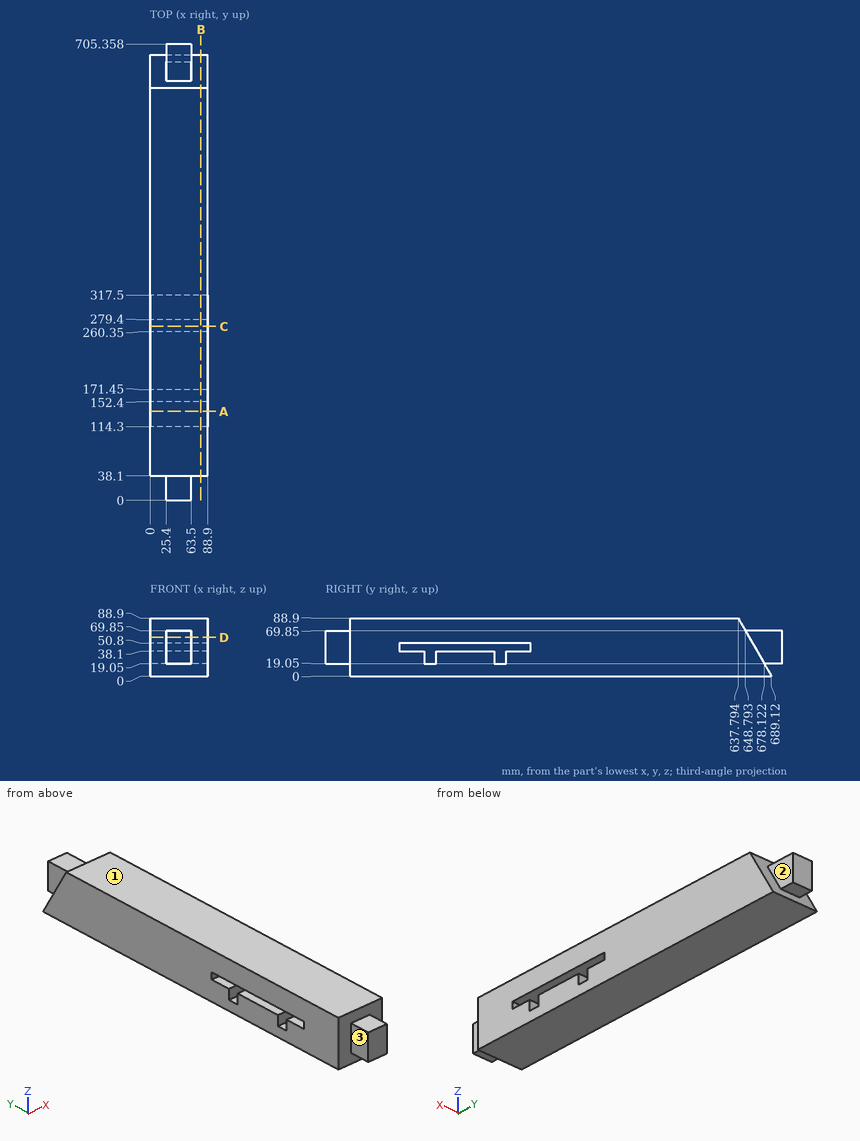
Geometry check sheet. Reference: drawing and pictorial views, mm from the part's lowest x, y, z. A direction names the side the tool comes from. Round coordinates to 2 decimals unless told otherwise and drop trailing zeros. Write each loop counter-clockwise with the first axis right and the second up, starting at its lowest first coordinate (ties: lowest second). Pieces come first, ordered by that corner, then holes. Notation, with made-up numbers: (-5.75, 34) -> (46.25, 34) arc R10 ccw to (46.25, 51) -> close; hole circle Ø4 at (-35, 2.5). An arc over 180 degrees is marked (long way). Put each result on its own line as item: value.
1) Cross-section at A-A, the plane y = 137.5. Enter the section's corners in (x, z), plus the area to 3 significant figures.
Recorded:
outline: (0, 0) -> (88.9, 0) -> (88.9, 38.1) -> (0, 38.1) -> close; (0, 50.8) -> (88.9, 50.8) -> (88.9, 88.9) -> (0, 88.9) -> close
area: 6,770 mm2
2) Cross-section at D-D, the plane z = 59.5. Enter the section's corners in (x, y).
Recorded:
outline: (0, 38.1) -> (25.4, 38.1) -> (25.4, 0) -> (63.5, 0) -> (63.5, 38.1) -> (88.9, 38.1) -> (88.9, 654.77) -> (63.5, 654.77) -> (63.5, 705.36) -> (25.4, 705.36) -> (25.4, 654.77) -> (0, 654.77) -> close
3) Cross-section at B-B, the plane x = 78.5. Enter the section's corners in (y, z).
Recorded:
outline: (38.1, 0) -> (689.12, 0) -> (637.79, 88.9) -> (38.1, 88.9) -> close; hole (114.3, 38.1) -> (152.4, 38.1) -> (152.4, 19.05) -> (171.45, 19.05) -> (171.45, 38.1) -> (260.35, 38.1) -> (260.35, 19.05) -> (279.4, 19.05) -> (279.4, 38.1) -> (317.5, 38.1) -> (317.5, 50.8) -> (114.3, 50.8) -> close
4) Access from +Z, -Z, +X, -X, +Y, -Y to the whole of each face (thin tool, end or side, straight path). Record for the marked faces 1, 2 and 3.
Recorded:
face 1: +Z, +X, -X, +Y, -Y
face 2: +Z, +X, +Y
face 3: +Z, -Z, -X, -Y
5) Cross-section at C-C, the plane y = 269. Enter the section's corners in (x, z).
Recorded:
outline: (0, 0) -> (88.9, 0) -> (88.9, 19.05) -> (0, 19.05) -> close; (0, 50.8) -> (88.9, 50.8) -> (88.9, 88.9) -> (0, 88.9) -> close
6) Thickness scan on probe 1 along Y at (x, z) = (53.5, 34.5); probe 2 along Z at (x, y) = (76, 180); probe 3 along Y at (x, z) = (11, 37). Record the ranges inside material, lowest first. Write a range as from..to.
Recorded:
probe 1: y = 0..152.4, 171.45..260.35, 279.4..705.36
probe 2: z = 0..38.1, 50.8..88.9
probe 3: y = 38.1..152.4, 171.45..260.35, 279.4..667.76
7) Depth check by flat-ended pin: P1, Ø21, axis at x = 57, z = 32, coming from the -Y side; P2, Ø6, axis at x = 12, z = 39.5, coming from the +Y side. Enter the tip coordinate at first touch or a pass-through.
Recorded:
P1: stops at y = 0
P2: stops at y = 668.05
